Part model, mm, in its own coordinate system. Face numbers are marked on the shaded views. A direction names the side the tool comes from. Round coordinates to 2 decimals unless told otherwise and drop trailing zeros. Order: outer loops, then holes, each group sorted by start corner. A loop starts at its lowest first (then second) coordinate and runs counter-clockwise, first axis right, second up. Notation, with made-up numbers: M 33.25,-17 L 91.25,-17 A13 cw 91.25,-2 Z; hole C 9,88 d10. An arc over 180 degrees is marked long. One line per question, with ' | ' between items.
from build123d import *

# Parameters (mm, degrees)
F0_W      = 150
F0_H      = 150
F1_DEPTH  = 33
F3_DEPTH  = 20
F4_R      = 5
F5_R      = 55
F6_DEPTH  = 30
F8_DEPTH  = 30
F9_R      = 52
F10_DEPTH = 83.001
F11_R     = 2.5
F12_DEPTH = 33.001
F13_R     = 2.5
F14_DEPTH = 33.001
F15_R     = 2.5
F16_DEPTH = 33.001
F17_R     = 2.5
F18_DEPTH = 33.001
F19_R     = 5
F20_R     = 2.5
F21_DEPTH = 75
F22_R     = 2.5
F23_DEPTH = 75


with BuildPart() as f1:
    # F0 (on Top) → F1 (new body)
    with BuildSketch(Plane.XY):
        with Locations((-0.500000082, -4.0026037022)):
            Rectangle(F0_W, F0_H)
    extrude(amount=F1_DEPTH)

    # F2 (on face) → F3 (join)
    with BuildSketch(Plane.XY.offset(33)):
        Polygon((24.499999918, 70.9973962978), (-25.500000082, 70.9973962978), (-75.500000082, 20.9973962978), (-75.500000082, -29.0026037022), (-25.500000082, -79.0026037022), (24.499999918, -79.0026037022), (74.499999918, -29.0026037022), (74.499999918, 20.9973962978), align=None)
    extrude(amount=F3_DEPTH)

    # F4
    f4_edges = [f1.edges().sort_by_distance(p)[0] for p in [
        (-75.5, 70.997396, 16.5),
        (-75.5, -79.002604, 16.5),
        (74.5, 70.997396, 16.5),
        (74.5, -79.002604, 16.5),
    ]]
    fillet(f4_edges, radius=F4_R)

    # F5 (on face) → F6 (join)
    with BuildSketch(Plane.XY.offset(53)):
        Circle(F5_R)
    extrude(amount=F6_DEPTH)

    # F7 (on face) → F8 (cut)
    with BuildSketch(Plane(origin=(0, 0, 0), x_dir=(1, 0, 0), z_dir=(0, 0, -1))):
        with BuildLine():
            Line((66.999999918, 76.5026037022), (-68.000000082, 76.5026037022))
            ThreePointArc((-68.000000082, 76.5026037022), (-71.5355339879, 75.0381376082), (-73.000000082, 71.5026037022))
            Line((-73.000000082, 71.5026037022), (-73.000000082, -63.4973962978))
            ThreePointArc((-73.000000082, -63.4973962978), (-71.5355339879, -67.0329302037), (-68.000000082, -68.4973962978))
            Line((-68.000000082, -68.4973962978), (66.999999918, -68.4973962978))
            ThreePointArc((66.999999918, -68.4973962978), (70.535533824, -67.0329302037), (71.999999918, -63.4973962978))
            Line((71.999999918, -63.4973962978), (71.999999918, 71.5026037022))
            ThreePointArc((71.999999918, 71.5026037022), (70.535533824, 75.0381376082), (66.999999918, 76.5026037022))
        make_face()
    extrude(amount=-F8_DEPTH, mode=Mode.SUBTRACT)

    # F9 (on face) → F10 (cut, through all)
    with BuildSketch(Plane.XY.offset(83)):
        Circle(F9_R)
    extrude(amount=-F10_DEPTH, mode=Mode.SUBTRACT)

    # F11 (on face) → F12 (cut, through all)
    with BuildSketch(Plane.XY.offset(33)):
        with Locations((-55.500000082, 50.9973962978)):
            Circle(F11_R)
    extrude(amount=-F12_DEPTH, mode=Mode.SUBTRACT)

    # F13 (on face) → F14 (cut, through all)
    with BuildSketch(Plane.XY.offset(33)):
        with Locations((54.499999918, 50.9973962978)):
            Circle(F13_R)
    extrude(amount=-F14_DEPTH, mode=Mode.SUBTRACT)

    # F15 (on face) → F16 (cut, through all)
    with BuildSketch(Plane.XY.offset(33)):
        with Locations((-55.500000082, -59.0026037022)):
            Circle(F15_R)
    extrude(amount=-F16_DEPTH, mode=Mode.SUBTRACT)

    # F17 (on face) → F18 (cut, through all)
    with BuildSketch(Plane.XY.offset(33)):
        with Locations((54.499999918, -59.0026037022)):
            Circle(F17_R)
    extrude(amount=-F18_DEPTH, mode=Mode.SUBTRACT)

    # F19
    f19_edges = [f1.edges().sort_by_distance(p)[0] for p in [
        (-75.5, -29.002604, 43),
        (-75.5, 20.997396, 43),
        (-25.5, -79.002604, 43),
        (24.5, -79.002604, 43),
        (74.5, -29.002604, 43),
        (74.5, 20.997396, 43),
        (24.5, 70.997396, 43),
        (-25.5, 70.997396, 43),
    ]]
    fillet(f19_edges, radius=F19_R)

    # F20 (on Right) → F21 (cut, symmetric)
    with BuildSketch(Plane.YZ):
        with Locations((0, 68)):
            Circle(F20_R)
    extrude(amount=F21_DEPTH, both=True, mode=Mode.SUBTRACT)

    # F22 (on Front) → F23 (cut, symmetric)
    with BuildSketch(Plane.XZ):
        with Locations((0, 68)):
            Circle(F22_R)
    extrude(amount=F23_DEPTH, both=True, mode=Mode.SUBTRACT)


solid = f1.part
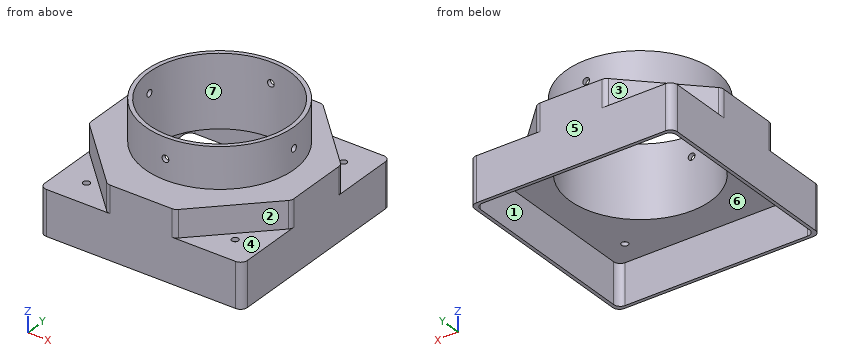
1) Saw through at B-B (z = 68). List the corners of the cut face in (x, y).
The answers:
outline: M -54.94,-2.5 A55 ccw -2.5,-54.94 L -2.5,-51.94 A52 cw -51.94,-2.5 Z; M -54.94,2.5 L -51.94,2.5 A52 cw -2.5,51.94 L -2.5,54.94 A55 ccw Z; M 2.5,-54.94 A55 ccw 54.94,-2.5 L 51.94,-2.5 A52 cw 2.5,-51.94 Z; M 2.5,51.94 A52 cw 51.94,2.5 L 54.94,2.5 A55 ccw 2.5,54.94 Z
2) Saw through at C-C (x = 31). List the corners of the cut face in (y, z).
The answers:
outline: M -79,0 L -76.5,0 L -76.5,30 L -41.75,30 L -41.75,83 L -45.43,83 L -45.43,53 L -72.5,53 L -72.5,33 L -79,33 Z; M 41.75,30 L 68.5,30 L 68.5,0 L 71,0 L 71,33 L 64.5,33 L 64.5,53 L 45.43,53 L 45.43,83 L 41.75,83 Z
3) Which spindle directions (+Z, -Z, +X, -X, +Y, -Y) get a long thin tool onto all of the face, cutting with end or side? Do the marked faces 1, 2 and 3. Say none if no direction does.
The answers:
face 1: -Z | face 2: +Z, +X, -Y | face 3: +Z, -X, +Y
4) Saw through at D-D (y = -39). List the corners of the cut face in (x, z), plus the area to 3 significant figures.
The answers:
outline: M -75.5,0 L -73,0 L -73,30 L -34.39,30 L -34.39,83 L -38.78,83 L -38.78,53 L -65.5,53 L -65.5,33 L -75.5,33 Z; M 34.39,30 L 72,30 L 72,0 L 74.5,0 L 74.5,33 L 64.5,33 L 64.5,53 L 38.78,53 L 38.78,83 L 34.39,83 Z | area: 1,880 mm²
5) Drop flat-ended pins along their axis: pin 1 (15.5 mm diameter, centred on x = -51, y = 43.5, fed in from +Z); pin 2 (12 mm diameter, centred on x = 23, z = 64, fed in from -Y); pin 3 (12 mm diameter, centred on x = -36.5, z = 59.5, fed in from +Y). Give the stop position or say it passes through.
The answers:
pin 1: stops at z = 53 | pin 2: stops at y = -52.31 | pin 3: stops at y = 45.77
6) Saw through at A-A (y = 0). List the corners of the cut face in (x, z), plus the area to 3 significant figures.
The answers:
outline: M -75.5,0 L -73,0 L -73,30 L -52,30 L -52,65.5 L -55,65.5 L -55,53 L -75.5,53 Z; M -55,70.5 L -52,70.5 L -52,83 L -55,83 Z; M 52,30 L 72,30 L 72,0 L 74.5,0 L 74.5,53 L 55,53 L 55,65.5 L 52,65.5 Z; M 52,70.5 L 55,70.5 L 55,83 L 52,83 Z | area: 1,360 mm²
7) Two-plate mould, pull along Y, no slides. Class the marked faces 4, 5, 6 and 7: released by +Y, released by -Y, zero draft, split by the parting line, or undercut.
The answers:
face 4: zero draft | face 5: released by +Y | face 6: undercut | face 7: undercut
8) Probe line 1 (Y direction, x = 20, z = 8); line 2 (Y direction, x = 0, z = 51); line 3 (Y direction, x = -55.5, z = 32.1). List the from-to ranges inside material, lowest first. Write a range as [from, to].
The answers:
line 1: y = [-79, -76.5], [68.5, 71] | line 2: y = [-79, -52], [52, 71] | line 3: y = [-79, -61.5], [-56.5, 48.5], [53.5, 71]
